Input: part model. Units: mm. Frame: model coordinates. Face numbers are marked on the shaded views. A direction names the side the tool comes from. Coordinates: 2 decimals unless noted, no trailing zeros. Order: outer loops, then holes, each group sorted by start corner. A loop starts at its lowest first (then second) coordinate and runs counter-clockwise, first axis right, second up. Notation, with made-up numbers: (31.5, -37) - (90.5, -37) arc R35 cw to (90.5, -2) - close; hole circle Ø9 at (-18.5, -8). An arc over 180 degrees is marked (long way). One line per question, with ' | ' between items. Start each with the question number.
```python
from build123d import *

# Parameters (mm, degrees)
SALIENTE_EXTRUIR1_DEPTH    = 40
CROQUIS5_W                 = 40
CROQUIS5_H                 = 10
CORTAR_EXTRUIR2_DEPTH      = 40
SALIENTE_EXTRUIR2_DEPTH    = 40
CROQUIS6_R                 = 2
CROQUIS6_W                 = 19
CROQUIS6_H                 = 42
CORTAR_EXTRUIR3_DEPTH      = 3
CORTAR_EXTRUIR3_DEPTH_BACK = 40
CROQUIS9_W                 = 6
CROQUIS9_H                 = 40
SALIENTE_EXTRUIR3_DEPTH    = 60
CROQUIS10_W                = 6
CROQUIS10_H                = 40
SALIENTE_EXTRUIR4_DEPTH    = 50
CROQUIS11_R                = 2.5
CORTAR_EXTRUIR4_DEPTH      = 1
CORTAR_EXTRUIR4_DEPTH_BACK = 93
CROQUIS12_W                = 80
CROQUIS12_H                = 6
SALIENTE_EXTRUIR5_DEPTH    = 40
CROQUIS13_W                = 19
CROQUIS13_H                = 20.4
CORTAR_EXTRUIR5_DEPTH      = 40
CROQUIS14_R                = 2
CROQUIS14_R_2              = 2.5
CORTAR_EXTRUIR6_DEPTH      = 40
REDONDEO3_R                = 5


with BuildPart() as part:
    # Croquis2 → Saliente-Extruir1 (new body)
    with BuildSketch(Plane.XY):
        Polygon((-31.145916957, -11.001243781), (-31.145916957, 23.998756219), (48.854083043, 23.998756219), (48.854083043, -11.001243781), (52.854083043, -11.001243781), (52.854083043, 27.998756219), (-35.145916957, 27.998756219), (-35.145916957, -11.001243781), align=None)
    extrude(amount=SALIENTE_EXTRUIR1_DEPTH)

    # Croquis5 → Cortar-Extruir2 (cut)
    with BuildSketch(Plane.ZY.offset(35.145916957)):
        with Locations((20, -6.001243781)):
            Rectangle(CROQUIS5_W, CROQUIS5_H)
    extrude(amount=-CORTAR_EXTRUIR2_DEPTH, mode=Mode.SUBTRACT)

    # Croquis7 → Saliente-Extruir2 (add)
    with BuildSketch(Plane.XY.offset(40)):
        Polygon((-35.145916957, -1.001243781), (-37.145916957, -1.001243781), (-37.145916957, 29.998756219), (54.854083043, 29.998756219), (54.854083043, -11.001243781), (52.854083043, -11.001243781), (52.854083043, 27.998756219), (-35.145916957, 27.998756219), align=None)
    extrude(amount=-SALIENTE_EXTRUIR2_DEPTH)

    # Croquis6 → Cortar-Extruir3 (cut, two sides)
    with BuildSketch(Plane(origin=(0, 27.998756219, 0), x_dir=(1, 0, 0), z_dir=(0, 1, 0))) as cortar_extruir3_sk:
        with Locations((13.854083043, -34)):
            Circle(CROQUIS6_R)
        with Locations((3.854083043, -34)):
            Circle(CROQUIS6_R)
        with Locations((-3.395916957, -29.25)):
            Circle(CROQUIS6_R)
        with Locations((-3.395916957, -19.25)):
            Circle(CROQUIS6_R)
        with Locations((21.104083043, -19.25)):
            Circle(CROQUIS6_R)
        with Locations((21.104083043, -29.25)):
            Circle(CROQUIS6_R)
        with Locations((8.854083043, -9)):
            Rectangle(CROQUIS6_W, CROQUIS6_H)
    extrude(amount=CORTAR_EXTRUIR3_DEPTH, mode=Mode.SUBTRACT)
    extrude(cortar_extruir3_sk.sketch, amount=-CORTAR_EXTRUIR3_DEPTH_BACK, mode=Mode.SUBTRACT)

    # Croquis9 → Saliente-Extruir3 (add)
    with BuildSketch(Plane.XZ.offset(1.001243781)):
        with Locations((-34.145916957, 20)):
            Rectangle(CROQUIS9_W, CROQUIS9_H)
    extrude(amount=SALIENTE_EXTRUIR3_DEPTH)

    # Croquis10 → Saliente-Extruir4 (add)
    with BuildSketch(Plane.XZ.offset(11.001243781)):
        with Locations((51.854083043, 20)):
            Rectangle(CROQUIS10_W, CROQUIS10_H)
    extrude(amount=SALIENTE_EXTRUIR4_DEPTH)

    # Croquis11 → Cortar-Extruir4 (cut, two sides)
    with BuildSketch(Plane.ZY.offset(37.145916957)) as cortar_extruir4_sk:
        with Locations((20, -46.001243781)):
            Circle(CROQUIS11_R)
    extrude(amount=CORTAR_EXTRUIR4_DEPTH, mode=Mode.SUBTRACT)
    extrude(cortar_extruir4_sk.sketch, amount=-CORTAR_EXTRUIR4_DEPTH_BACK, mode=Mode.SUBTRACT)

    # Croquis12 → Saliente-Extruir5 (add)
    with BuildSketch(Plane.XZ.offset(-23.998756219)):
        with Locations((8.854083043, 3)):
            Rectangle(CROQUIS12_W, CROQUIS12_H)
    extrude(amount=SALIENTE_EXTRUIR5_DEPTH)

    # Croquis13 → Cortar-Extruir5 (cut)
    with BuildSketch(Plane(origin=(0, 0, 0), x_dir=(-1, 0, 0), z_dir=(0, 0, -1))):
        with Locations((-8.854083043, 13.798756219)):
            Rectangle(CROQUIS13_W, CROQUIS13_H)
    extrude(amount=-CORTAR_EXTRUIR5_DEPTH, mode=Mode.SUBTRACT)

    # Croquis14 → Cortar-Extruir6 (cut)
    with BuildSketch(Plane.ZY.offset(37.145916957)):
        with Locations((25, -51.001243781)):
            Circle(CROQUIS14_R)
        with Locations((25, -41.001243781)):
            Circle(CROQUIS14_R)
        with Locations((15, -51.001243781)):
            Circle(CROQUIS14_R)
        with Locations((15, -41.001243781)):
            Circle(CROQUIS14_R)
        with Locations((20, -46.001243781)):
            Circle(CROQUIS14_R_2)
    extrude(amount=-CORTAR_EXTRUIR6_DEPTH, mode=Mode.SUBTRACT)

    # Redondeo3
    redondeo3_edges = [part.edges().sort_by_distance(p)[0] for p in [
        (-37.145916957, -15.501243781, 0),
        (54.854083043, -15.501243781, 0),
    ]]
    fillet(redondeo3_edges, radius=REDONDEO3_R)


solid = part.part
```
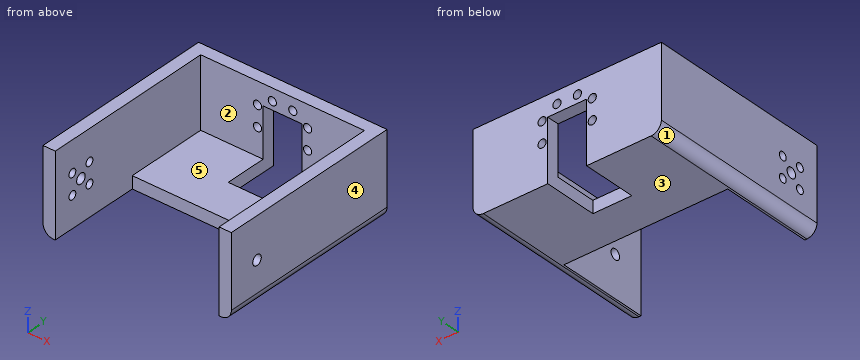
(1) Section B-B (z = 25). Output: boundary loops of the cut face in (x, y).
(2) Reachability of the marked faces 1 and 2 from +Z, -Z, +X, -X, +Y, -Y: full face, straight path, thin tool, end or side. Return the list, or none.
(3) Section A-A (z = 34). Output: boundary loops of the cut face in (x, y).
(4) Section C-C (y = 1). Output: boundary loops of the cut face in (x, z).
(5) Material intervals for line 1 along X through (y, z) = (26, 34); line 2 along X through (y, z) = (16.5, 36.5); line 3 along Y through (x, z) = (-33, 20), sorted ascending. Write a range as from..to.
(6) Section D-D (y = 16). Output: boundary loops of the cut face in (x, z).
(7) Draft query along X for the marked faces 3, 4 and 5. Return one class per face: +X half, -X half, draft (parallel to the pull), parting line (faces both ways), or undercut.
(8) Pin query (flat end, axial travel): pin 1 (3 mm diameter, centred on x = 12, y = 27, fed in from -Z); pin 2 (12 mm diameter, centred on x = 10.5, z = 5, fed in from -Y); pin 3 (3.5 mm diameter, centred on x = -3.4, z = 29.25, fed in from +Y); pin 4 (10 mm diameter, centred on x = 3.5, z = 29.5, fed in from -Y). Return the tip coordinate at first contact, or that it passes through.
Worked answers:
1) outline: (-37.15, -61) - (-31.15, -61) - (-31.15, -53) - (-37.15, -53) - close; (-37.15, -49) - (-31.15, -49) - (-31.15, -43) - (-37.15, -43) - close; (-37.15, -39) - (-31.15, -39) - (-31.15, 24) - (-0.65, 24) - (-0.65, 30) - (-37.15, 30) - close; (18.35, 24) - (48.85, 24) - (48.85, -61) - (54.85, -61) - (54.85, 30) - (18.35, 30) - close
2) face 1: -Z, -X, +Y, -Y | face 2: +Z, -Y
3) outline: (-37.15, -61) - (-31.15, -61) - (-31.15, 24) - (1.85, 24) - (1.85, 30) - (-37.15, 30) - close; (5.85, 24) - (11.85, 24) - (11.85, 30) - (5.85, 30) - close; (15.85, 24) - (48.85, 24) - (48.85, -61) - (54.85, -61) - (54.85, 30) - (15.85, 30) - close
4) outline: (-37.15, 5) arc R5 ccw to (-32.15, 0) - (49.85, 0) arc R5 ccw to (54.85, 5) - (54.85, 40) - (48.85, 40) - (48.85, 6) - (-31.15, 6) - (-31.15, 40) - (-37.15, 40) - close
5) line 1: x = -37.15..1.85, 5.85..11.85, 15.85..54.85 | line 2: x = -37.15..-31.15, 48.85..54.85 | line 3: y = -61..-48.5, -43.5..30
6) outline: (-37.15, 5) arc R5 ccw to (-32.15, 0) - (-0.65, 0) - (-0.65, 6) - (-31.15, 6) - (-31.15, 40) - (-37.15, 40) - close; (18.35, 0) - (49.85, 0) arc R5 ccw to (54.85, 5) - (54.85, 40) - (48.85, 40) - (48.85, 6) - (18.35, 6) - close
7) face 3: draft | face 4: +X half | face 5: undercut
8) pin 1: stops at z = 30 | pin 2: stops at y = -16 | pin 3: passes through | pin 4: stops at y = 24
